Geometry: see drawing. Coordinates: mm, zero at the bounding-box minimum. A direction names the side the tool comes from. Coordinates: 2 decimals unless noted, no trailing zeros. Loops run counter-clockwise (first coordinate to the right, second up) from the corner with the lowest first, then second, coordinate; pieces in that order, holes last. Notation, with made-up numbers: (10, 86) -> (61, 86) arc R20 ccw to (61, 108) -> close; hole circle Ø1 at (-24.5, 22). An arc over 180 degrees is marked (long way). One line per item, written item: value. Start each with the question number.
Item 1: Ray query, probe 1 along X at (y, z) = (19, 20); probe 2 along X at (y, z) = (11, 8.5); probe 3 along Y at (x, z) = (57, 26.5) (1 decimal). Return the intervals inside material, ascending. Write a range as from..to.
Item 2: Set-up query: the marked faces 1, 2 and 3. Return all of +Z, -Z, +X, -X, +Y, -Y with unobstructed straight access to the full face (end or side cutting, diameter ignored); none if empty.
Item 3: Mould query, pull axis X, two halves, no side actions, for the marked faces 4, 5, 6 and 7. Classes: +X half, -X half, draft (parallel to the pull), parting line (faces both ways), or undercut.
Item 4: Section query D-D on x = 29.5. Return loops of the section in (y, z) (1 decimal).
Item 5: Contact query for flat-ended pins moving along their axis: pin 1 Ø6.5 at (x, y) = (46, 15) entering from -Z; pin 2 Ø1 at (y, z) = (17, 32) entering from +X; pin 3 Ø1 at (x, y) = (56.5, 19.5) entering from -Z. Output: stop coordinate, or through.
Item 6: Section query B-B on z = 15. Return loops of the section in (x, y), then the cut area to 3 significant figures.
Item 7: Section query A-A on x = 57.15. Return loops of the section in (y, z) (1 decimal).
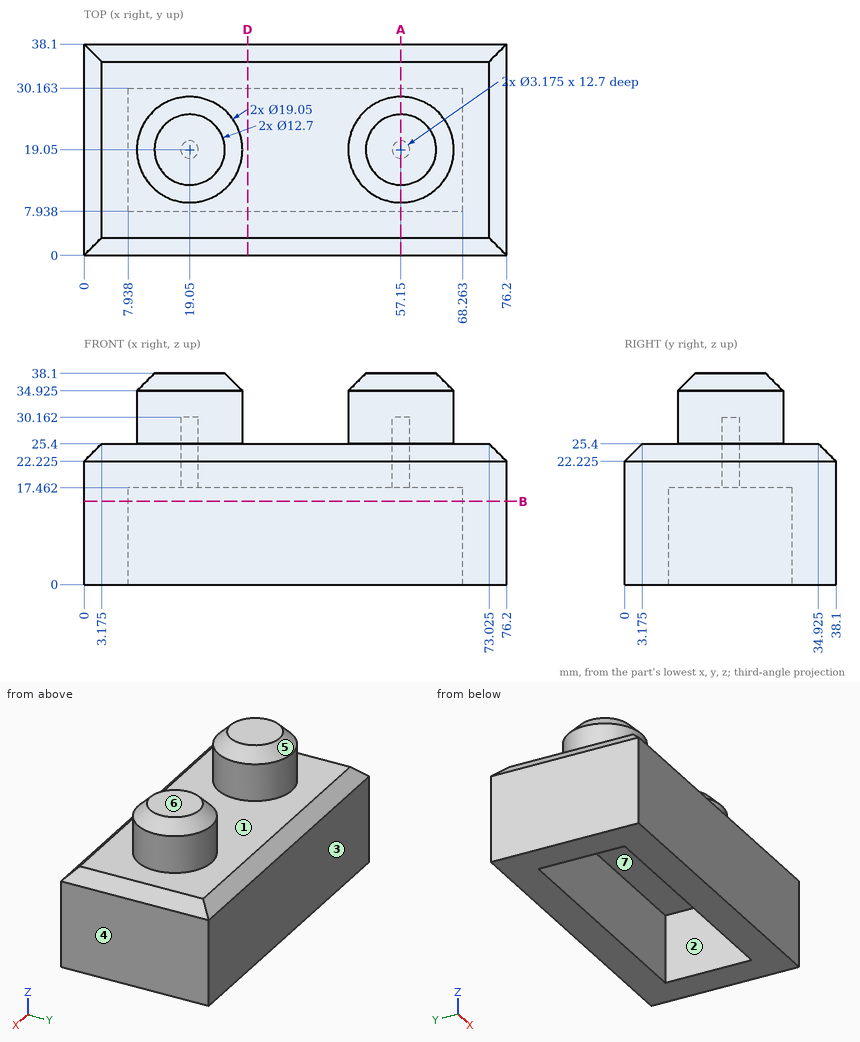
Reply:
1. probe 1: x = 0..17.46, 20.64..55.56, 58.74..76.2
1. probe 2: x = 0..7.94, 68.26..76.2
1. probe 3: y = 9.5..17.5, 20.6..28.6
2. face 1: +Z
2. face 2: -Z
2. face 3: +Z, -Z, +X, -X, +Y
3. face 4: +X half
3. face 5: undercut
3. face 6: draft
3. face 7: undercut
4. outline: (0, 0) -> (7.9, 0) -> (7.9, 17.5) -> (30.2, 17.5) -> (30.2, 0) -> (38.1, 0) -> (38.1, 22.2) -> (34.9, 25.4) -> (3.2, 25.4) -> (0, 22.2) -> close
5. pin 1: stops at z = 17.46
5. pin 2: stops at x = 66.55
5. pin 3: stops at z = 30.16
6. outline: (0, 0) -> (76.2, 0) -> (76.2, 38.1) -> (0, 38.1) -> close; hole (7.94, 7.94) -> (68.26, 7.94) -> (68.26, 30.16) -> (7.94, 30.16) -> close
6. area: 1,560 mm²
7. outline: (0, 0) -> (7.9, 0) -> (7.9, 17.5) -> (17.5, 17.5) -> (17.5, 30.2) -> (20.6, 30.2) -> (20.6, 17.5) -> (30.2, 17.5) -> (30.2, 0) -> (38.1, 0) -> (38.1, 22.2) -> (34.9, 25.4) -> (28.6, 25.4) -> (28.6, 34.9) -> (25.4, 38.1) -> (12.7, 38.1) -> (9.5, 34.9) -> (9.5, 25.4) -> (3.2, 25.4) -> (0, 22.2) -> close
